```python
from build123d import *

# Parameters (mm, degrees)
F0_R     = 4.5
F1_DEPTH = 88
F2_R     = 4
F3_DEPTH = 25
F4_R     = 10
F4_R_2   = 4.5
F5_DEPTH = 5


# Not quite as in the source:
# - a fillet or chamfer that OpenCascade refuses, or shapes differently, is made with other operations: its cross-section is extruded or revolved along the edge and cut away or added


with BuildPart() as f1:
    # F0 (on Front) → F1 (new body)
    with BuildSketch(Plane.XZ):
        Circle(F0_R)
    extrude(amount=F1_DEPTH)

    # F2 (on face) → F3 (cut)
    with BuildSketch(Plane.XZ.offset(88)):
        Circle(F2_R)
    extrude(amount=-F3_DEPTH, mode=Mode.SUBTRACT)

    # F4 (on face) → F5 (join)
    with BuildSketch(Plane(origin=(0, 0, 0), x_dir=(-1, 0, 0), z_dir=(0, 1, 0))):
        Circle(F4_R)
        Circle(F4_R_2, mode=Mode.SUBTRACT)
        Circle(F4_R_2)
    extrude(amount=F5_DEPTH)

    # F6: fillet of radius 10 on 1 edges, made by hand

    # F6_s1 → F6_t2 (revolve, cut)
    with BuildSketch(Plane.XY):
        with BuildLine():
            ThreePointArc((-10, 0), (-6.3397459622, 3.6602540378), (-1.3397459622, 5))
            Line((-1.3397459622, 5), (-10, 5))
            Line((-10, 5), (-10, 0))
        make_face()
    revolve(axis=Axis((0, 5, 0), (0, 1, 0)), mode=Mode.SUBTRACT)


solid = f1.part
```
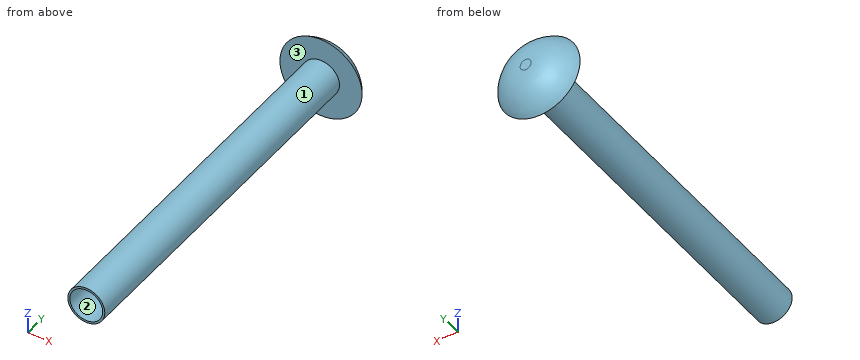
Work out the finished part from the listing and answer in its coordinate system (mm). Face numbers are marked on the shaded views. Give positions to 0.01 mm unless a question says otherwise; leave off trailing zeros. Write each loop counter-clockwise with the first axis right and the second up, starting at its lowest first coordinate (ties: lowest second). Pieces come first, ordered by that corner, then holes. Notation, with made-up numbers: (42.5, -32) -> (89.5, -32) arc R17 ccw to (89.5, -22) -> close; hole circle Ø2 at (8.25, 19.5). An arc over 180 degrees is marked (long way). Write item = value, one per line.
Q1. Consider line 1 along Z through (x, y) = (0, -71); line 2 along Z through (x, y) = (2.5, -74); line 3 along X through (y, z) = (-76.5, 0.25). Determine where each line is inside the solid, lowest interval first.
Computed values:
line_1 = -4.5 to -4, 4 to 4.5
line_2 = -3.74 to -3.12, 3.12 to 3.74
line_3 = -4.49 to -3.99, 3.99 to 4.49
Q2. Flat-ended cylindrical pins translate along their axes: pin 1 Ø1 at (y, z) = (-23.5, 3) entering from +X; pin 2 Ø12 at (y, z) = (-73.5, 3.5) entering from -X; pin 3 Ø1.5 at (y, z) = (-10.5, -7) entering from +X; pin 4 Ø10 at (y, z) = (-63, 2) entering from +X. Find the tip coordinate at first contact, or state that the pin passes through.
Computed values:
pin_1 = 3.74
pin_2 = -4.5
pin_3 = through
pin_4 = 4.5
Q3. Section A-A on y = -66 is taken. Determine the outline of the cut face in (x, z).
Computed values:
outline = circle Ø9 at (0, 0); hole circle Ø8 at (0, 0)
Q4. Section B-B on y = -21 is taken. Determine the outline of the cut face in (x, z).
Computed values:
outline = circle Ø9 at (0, 0)
Q5. For a pull along X with two mould halves and no side action, classify the marked faces 1, 2 and 3 as pulls with the +X half, pulls with the -X half, needs draft (parallel to the pull), parting line crosses it, or undercut.
Computed values:
face_1 = parting line crosses it
face_2 = undercut
face_3 = needs draft
